from build123d import *

# Parameters (mm, degrees)
SKETCH_R        = 2.65
PAD_DEPTH       = 4
SKETCH001_W     = 7
SKETCH001_H     = 1.2
SKETCH001_W_2   = 8
POCKET_DEPTH    = 60.001
SKETCH002_W     = 7
SKETCH002_H     = 1.2
SKETCH002_W_2   = 8
POCKET001_DEPTH = 60.001


with BuildPart() as part:
    # Sketch → Pad (new body)
    with BuildSketch(Plane.XY):
        Polygon((0, 0), (0, 60), (-20, 60), (-60, 20), (-60, 0), align=None)
        with Locations((-50, 10)):
            Circle(SKETCH_R, mode=Mode.SUBTRACT)
        with Locations((-10, 10)):
            Circle(SKETCH_R, mode=Mode.SUBTRACT)
        with Locations((-30, 10)):
            Circle(SKETCH_R, mode=Mode.SUBTRACT)
        with Locations((-10, 50)):
            Circle(SKETCH_R, mode=Mode.SUBTRACT)
        with Locations((-10, 30)):
            Circle(SKETCH_R, mode=Mode.SUBTRACT)
    extrude(amount=PAD_DEPTH)

    # Sketch001 → Pocket (cut, through all)
    with BuildSketch(Plane.XZ):
        with Locations((-3.5, 3.4)):
            Rectangle(SKETCH001_W, SKETCH001_H)
        with Locations((-17, 3.4)):
            Rectangle(SKETCH001_W_2, SKETCH001_H)
    extrude(amount=-POCKET_DEPTH, mode=Mode.SUBTRACT)

    # Sketch002 → Pocket001 (cut, through all)
    with BuildSketch(Plane.YZ):
        with Locations((3.5, 3.4)):
            Rectangle(SKETCH002_W, SKETCH002_H)
        with Locations((17, 3.4)):
            Rectangle(SKETCH002_W_2, SKETCH002_H)
    extrude(amount=-POCKET001_DEPTH, mode=Mode.SUBTRACT)


solid = part.part
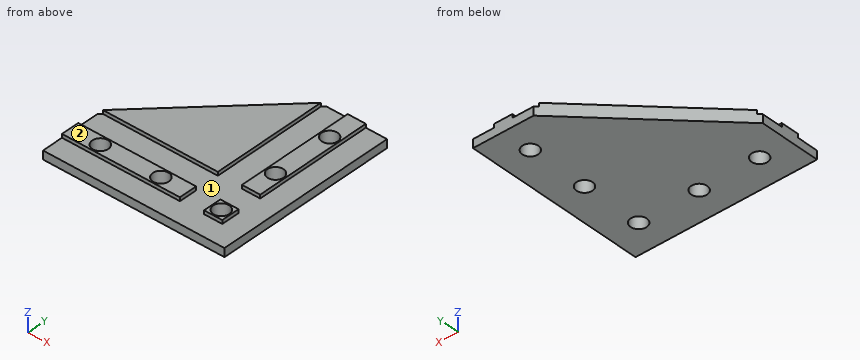
Model file for the job. Use its own axes, mm. Face numbers are marked on the shaded views. Give positions to 0.01 mm unless a question says otherwise; leave off trailing zeros. Loops run counter-clockwise (first coordinate to the right, second up) from the corner with the lowest first, then second, coordinate; pieces in that order, holes last.
1) Saw through at D-D (y = 30). Write the cut outline in (x, z).
2) Saw through at A-A (y = 10). Write the cut outline in (x, z), plus the area to 3 significant figures.
3) Wall check: line 1 (Y direction, x = -10, z = 3.2); line 2 (Y direction, x = -10, z = 2.05); line 3 (Y direction, x = -8, z = 2). Give the ranges that are in metal, low to high.
4) Pull direction Y, two halves, no side cores. Call the marked faces 1 and 2: +Y half, -Y half, draft (parallel to the pull), parting line (faces both ways), or undercut.
5) Saw through at B-B (x = -30). Write the cut outline in (y, z).
6) Flat gauge pins, fed straight in: pin 1 Ø1 at (x, z) = (-52, 1.5) entering from +Y; pin 2 Ø1.3 at (y, z) = (46.5, 3) entering from +X; pin 3 Ø1 at (y, z) = (33.5, 3.5) entering from +X; pin 4 Ø1.3 at (y, z) = (44.5, 3.5) entering from -X. Where does each tip first touch, or does it go through?
7) Saw through at C-C (z = 1.85). Write the cut outline in (x, y), plus the area to 3 significant figures.
Answer block:
1. outline: (-50, 0) - (-12.65, 0) - (-12.65, 4) - (-13, 4) - (-13, 2.8) - (-21, 2.8) - (-21, 4) - (-50, 4) - close; (-7.35, 0) - (0, 0) - (0, 2.8) - (-7, 2.8) - (-7, 4) - (-7.35, 4) - close
2. outline: (-60, 0) - (-52.65, 0) - (-52.65, 4) - (-60, 4) - close; (-47.35, 0) - (-32.65, 0) - (-32.65, 4) - (-47.35, 4) - close; (-27.35, 0) - (-12.65, 0) - (-12.65, 4) - (-13, 4) - (-13, 2.8) - (-21, 2.8) - (-21, 4) - (-27.35, 4) - close; (-7.35, 0) - (0, 0) - (0, 2.8) - (-7, 2.8) - (-7, 4) - (-7.35, 4) - close
2. area: 158 mm2
3. line 1: y = 7 to 7.35, 12.65 to 13, 21 to 27.35, 32.65 to 47.35, 52.65 to 60
3. line 2: y = 0 to 7.35, 12.65 to 27.35, 32.65 to 47.35, 52.65 to 60
3. line 3: y = 0 to 8.26, 11.74 to 28.26, 31.74 to 48.26, 51.74 to 60
4. face 1: undercut
4. face 2: draft
5. outline: (0, 0) - (7.35, 0) - (7.35, 4) - (7, 4) - (7, 2.8) - (0, 2.8) - close; (12.65, 0) - (50, 0) - (50, 4) - (21, 4) - (21, 2.8) - (13, 2.8) - (13, 4) - (12.65, 4) - close
6. pin 1: stops at y = 28.5
6. pin 2: stops at x = 0
6. pin 3: stops at x = -7
6. pin 4: stops at x = -36.15
7. outline: (-60, 0) - (0, 0) - (0, 60) - (-20, 60) - (-60, 20) - close; hole circle Ø5.3 at (-50, 10); hole circle Ø5.3 at (-30, 10); hole circle Ø5.3 at (-10, 10); hole circle Ø5.3 at (-10, 30); hole circle Ø5.3 at (-10, 50)
7. area: 2,690 mm2
